```python
from build123d import *

# Parameters (mm, degrees)
SKETCH1_R           = 1.778
BOSS_EXTRUDE1_DEPTH = 3.175
SKETCH2_W           = 38.1
SKETCH2_H           = 9.525
CUT_EXTRUDE1_DEPTH  = 105.692755002
FILLET1_R           = 2.54
SKETCH3_R           = 6.35
CUT_EXTRUDE2_DEPTH  = 105.692755002
SKETCH4_W           = 3.175
SKETCH4_H           = 109.22
BOSS_EXTRUDE2_DEPTH = 3.175


with BuildPart() as part:
    # Sketch1 → Boss-Extrude1 (new body)
    with BuildSketch(Plane.XY):
        Polygon((-89.265, -54.61), (59.69, -54.61), (59.69, 54.61), (-89.265, 54.61), (-89.265, 9.935), align=None)
        with Locations((-52.715, -47.635)):
            Circle(SKETCH1_R, mode=Mode.SUBTRACT)
        with Locations((52.715, -47.635)):
            Circle(SKETCH1_R, mode=Mode.SUBTRACT)
        with Locations((-52.715, 47.635)):
            Circle(SKETCH1_R, mode=Mode.SUBTRACT)
        with Locations((52.715, 47.635)):
            Circle(SKETCH1_R, mode=Mode.SUBTRACT)
    extrude(amount=BOSS_EXTRUDE1_DEPTH)

    # Sketch2 → Cut-Extrude1 (cut, through all)
    with BuildSketch(Plane.XY.offset(3.175)):
        with Locations((27.315, -42.8725)):
            Rectangle(SKETCH2_W, SKETCH2_H)
    extrude(amount=-CUT_EXTRUDE1_DEPTH, mode=Mode.SUBTRACT)

    # Fillet1
    fillet1_edges = [part.edges().sort_by_distance(p)[0] for p in [
        (46.365, -47.635, 1.5875),
        (8.265, -47.635, 1.5875),
        (8.265, -38.11, 1.5875),
        (46.365, -38.11, 1.5875),
    ]]
    fillet(fillet1_edges, radius=FILLET1_R)

    # Sketch3 → Cut-Extrude2 (cut, through all)
    with BuildSketch(Plane.XY.offset(3.175)):
        with Locations((-52.715, 0)):
            Circle(SKETCH3_R)
    extrude(amount=-CUT_EXTRUDE2_DEPTH, mode=Mode.SUBTRACT)

    # Sketch4 → Boss-Extrude2 (add)
    with BuildSketch(Plane.ZY.offset(89.265)):
        with Locations((1.5875, 0)):
            Rectangle(SKETCH4_W, SKETCH4_H)
    extrude(amount=BOSS_EXTRUDE2_DEPTH)


solid = part.part
```
The listing builds one solid part. Answer for the finished solid, in the listing's coordinates (mm). A direction names the side the tool comes from. Coordinates: 2 decimals unless noted, no trailing zeros. Write each loop counter-clockwise with the first axis right and the second up, starting at its lowest first coordinate (ties: lowest second). Pieces come first, ordered by that corner, then holes. Notation, with made-up numbers: (33, 50.25) - (72, 50.25) arc R26 cw to (72, 73.25) - close; hole circle Ø11 at (-14.5, 28). An arc over 180 degrees is marked (long way). One line per item, written item: value.
1) For a pull along Y with two mould halves and no side action, classify faces 3 (the flat face through (-15, 54.61, 2)), 4 (the flat face through (59.69, -1, 2)), 5 (the flat face through (27, -38.11, 2)), 6 (the cylindrical face through (51.304, 46.553, 1.565)) as pulls with the +Y half, pulls with the -Y half, needs draft (parallel to the pull), parting line crosses it, or undercut.
Geometry check:
face 3: pulls with the +Y half
face 4: needs draft
face 5: undercut
face 6: undercut
2) Find section A-A (x = 34.5). Give the vertices of the cut face in (y, z) (3 decimals), and give its area (3 significant figures).
Geometry check:
outline: (-54.61, 0) - (-47.635, 0) - (-47.635, 3.175) - (-54.61, 3.175) - close; (-38.11, 0) - (54.61, 0) - (54.61, 3.175) - (-38.11, 3.175) - close
area: 317 mm2
3) A tool of negligible diameter and unlimited length cuts with its end or side. For faces 1 (the flat face through (-92.44, 1, 2)), 2 (the flat face through (27, -47.635, 2)), from which of +Z, -Z, +X, -X, +Y, -Y can it reach the whole face along a straight path? Write none if from no direction.
Geometry check:
face 1: +Z, -Z, -X, +Y, -Y
face 2: +Z, -Z
4) Find section C-C (z = 0.7). Give the vertices of the cut face in (x, y) (3 decimals), and give its area (3 significant figures).
Geometry check:
outline: (-92.44, -54.61) - (59.69, -54.61) - (59.69, 54.61) - (-92.44, 54.61) - close; hole circle Ø12.7 at (-52.715, 0); hole circle Ø3.556 at (-52.715, -47.635); hole circle Ø3.556 at (-52.715, 47.635); hole (8.265, -45.095) arc R2.54 ccw to (10.805, -47.635) - (43.825, -47.635) arc R2.54 ccw to (46.365, -45.095) - (46.365, -40.65) arc R2.54 ccw to (43.825, -38.11) - (10.805, -38.11) arc R2.54 ccw to (8.265, -40.65) - close; hole circle Ø3.556 at (52.715, -47.635); hole circle Ø3.556 at (52.715, 47.635)
area: 16,100 mm2
5) Consider line 1 along Y through (x, z) = (20, 1.55) (3 decimals); line 2 along Y through (x, z) = (53, 2.45); line 3 along X through (y, z) = (-46.5, 0.35). Determine where each line is inside the solid, lowest interval first. Write a range as from..to.
Geometry check:
line 1: y = -54.61..-47.635, -38.11..54.61
line 2: y = -54.61..-49.39, -45.88..45.88, 49.39..54.61
line 3: x = -92.44..-54.08, -51.35..8.69, 45.94..51.35, 54.08..59.69
6) Find section B-B (y = 0). Give the vertices of the cut face in (x, z) (3 decimals).
Geometry check:
outline: (-92.44, 0) - (-59.065, 0) - (-59.065, 3.175) - (-92.44, 3.175) - close; (-46.365, 0) - (59.69, 0) - (59.69, 3.175) - (-46.365, 3.175) - close
